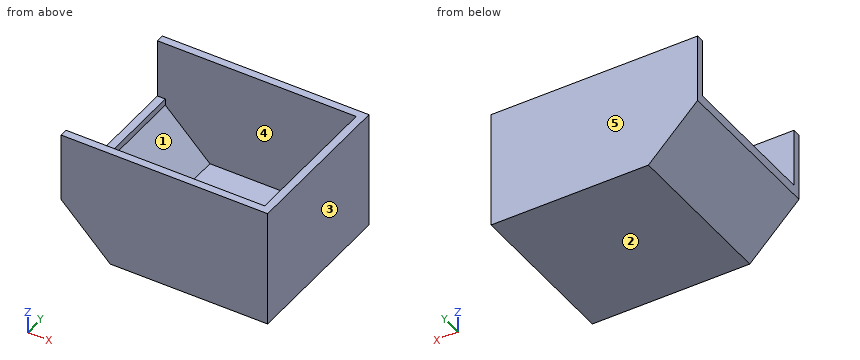
from build123d import *

# Parameters (mm, degrees)
F0_W     = 133.35
F0_H     = 104.775
F1_DEPTH = 76.2
F2_SIZE  = 31.75
F3_T     = -5.08
F4_W     = 94.615
F4_H     = 38.1
F5_DEPTH = 25.4


with BuildPart() as f1:
    # F0 (on Top) → F1 (new body)
    with BuildSketch(Plane.XY):
        with Locations((66.675, 52.3875)):
            Rectangle(F0_W, F0_H)
    extrude(amount=F1_DEPTH)

    # F2
    f2_edges = [f1.edges().sort_by_distance(p)[0] for p in [
        (0, 52.3875, 0),
    ]]
    chamfer(f2_edges, length=F2_SIZE)

    # F3
    f3_openings = [f1.faces().sort_by_distance(p)[0] for p in [
        (66.675, 52.3875, 76.2),
    ]]
    offset(amount=F3_T, openings=f3_openings)

    # F4 (on face) → F5 (cut)
    with BuildSketch(Plane.YZ.offset(5.08)):
        with Locations((52.3875, 57.15)):
            Rectangle(F4_W, F4_H)
    extrude(amount=-F5_DEPTH, mode=Mode.SUBTRACT)


solid = f1.part
Could you check a few things on this model? Use its own coordinates, in mm. Face numbers are marked on the shaded views. A direction names the side the tool comes from. Give positions to 0.01 mm unless a question says otherwise; leave off trailing zeros. Order: outer loops, then holes, each group sorted by start corner. A loop starts at its lowest first (then second) coordinate and runs counter-clockwise, first axis right, second up. Notation, with made-up numbers: (35, 27) - (80, 27) arc R27 ccw to (80, 51) - close; hole circle Ø3 at (85, 81.5). An arc over 180 degrees is marked (long way). One line per question, with ' | ' between items. Start each with the question number.
Item 1: I want a section at A-A on z = 69. Write out the boundary of the cut face in (x, y) (3 decimals), then the cut area to 3 significant figures.
Item 2: I'm going to push flat-ended pins straight in: pin 1 Ø3 at (y, z) = (65, 58) entering from -X; pin 2 Ø5 at (x, y) = (41.5, 59) entering from +Z; pin 3 Ø5.5 at (x, y) = (3.5, 73) entering from +Z. Where does each tip first touch, or does it pass through?
Item 3: I want a section at D-D on z = 36. Write out the boundary of the cut face in (x, y) (3 decimals).
Item 4: Thinking about a two-plate mould opening in X: for the marked faces 3, 4 and 5, which applies, pulls with the +X half, pulls with the -X half, needs draft (parallel to the pull), parting line crosses it, or undercut?
Item 5: I want a section at C-C on x = 35.5. Write out the boundary of the cut face in (y, z) (3 decimals).
Item 6: For the marked faces 1 and 2, which set-ups out of +Z, -Z, +X, -X, +Y, -Y let a thin tool reach every point of the face, with its end or its side?
Item 7: I want a section at B-B on y = 31. Write out the boundary of the cut face in (x, z).
Item 8: I need wall thicknesses on probe 1 along Y at (x, z) = (18, 40) (3 decimals); probe 2 along X at (y, z) = (93.5, 35.5); probe 3 along X at (y, z) = (9, 15.5). Which ranges of each line are inside material? Lowest first, please. Write a range as [from, to].
Verdict:
1) outline: (0, 0) - (133.35, 0) - (133.35, 104.775) - (0, 104.775) - (0, 99.695) - (128.27, 99.695) - (128.27, 5.08) - (0, 5.08) - close | area: 1,840 mm^2
2) pin 1: x = 128.27 | pin 2: z = 5.08 | pin 3: z = 38.1
3) outline: (0, 0) - (133.35, 0) - (133.35, 104.775) - (0, 104.775) - close; hole (5.08, 5.08) - (128.27, 5.08) - (128.27, 99.695) - (5.08, 99.695) - close
4) face 3: pulls with the +X half | face 4: undercut | face 5: needs draft
5) outline: (0, 0) - (104.775, 0) - (104.775, 76.2) - (99.695, 76.2) - (99.695, 5.08) - (5.08, 5.08) - (5.08, 76.2) - (0, 76.2) - close
6) face 1: +Z | face 2: -Z, +X, -X, +Y, -Y
7) outline: (0, 31.75) - (31.75, 0) - (133.35, 0) - (133.35, 76.2) - (128.27, 76.2) - (128.27, 5.08) - (33.85, 5.08) - (5.08, 33.85) - (5.08, 38.1) - (0, 38.1) - close
8) probe 1: [0, 5.08], [99.695, 104.775] | probe 2: [0, 5.08], [128.27, 133.35] | probe 3: [16.25, 23.43], [128.27, 133.35]
